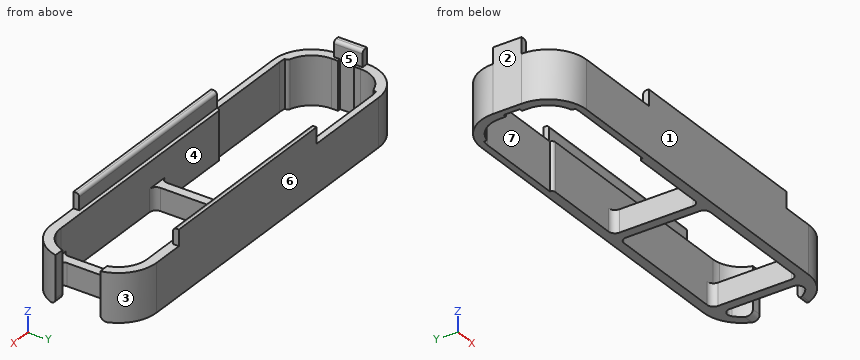
from build123d import *

# Parameters (mm, degrees)
BOSS_EXTRUDE2_DEPTH                    = 15
SKETCH4_W                              = 3
SKETCH4_H                              = 27
BOSS_EXTRUDE4_CROSS_STRUCTURES_DEPTH   = 15
SKETCH6_W                              = 3
SKETCH6_H                              = 27
CUT_EXTRUDE3_8_MM_SPACING_DEPTH        = 8
CUT_EXTRUDE4_ELECTRONICS_SPACING_DEPTH = 125.021167548
SKETCH8_W                              = 15
SKETCH8_H                              = 14
CUT_EXTRUDE2_USB_C_CUTOUT_DEPTH        = 5
FILLET2_USBC_R                         = 2
FILLET3_INNER_CORNERS_FRONT_R          = 1
FILLET5_INNER_CORNERS_R                = 2
SKETCH18_W                             = 62
SKETCH18_H                             = 1.8
SKETCH18_W_2                           = 2
SKETCH18_H_2                           = 9
BOSS_EXTRUDE7_DEPTH                    = 5
FILLET1_R                              = 1
SKETCH19_W                             = 1
SKETCH19_H                             = 5
CUT_EXTRUDE1_DEPTH                     = 124.762162398


with BuildPart() as part:
    # Sketch3 → Boss-Extrude2 (new body)
    with BuildSketch(Plane.XY.offset(-1.6194024)):
        with BuildLine():
            Line((110, 16.5), (10, 16.5))
            ThreePointArc((10, 16.5), (1.514718626, 12.985281374), (-2, 4.5))
            Line((-2, 4.5), (-2, -4.5))
            ThreePointArc((-2, -4.5), (1.514718626, -12.985281374), (10, -16.5))
            Line((10, -16.5), (110, -16.5))
            ThreePointArc((110, -16.5), (118.485281374, -12.985281374), (122, -4.5))
            Line((122, -4.5), (122, 4.5))
            ThreePointArc((122, 4.5), (118.485281374, 12.985281374), (110, 16.5))
        make_face()
        with BuildLine():
            Line((119, -4.5), (119, 4.5))
            ThreePointArc((119, 4.5), (116.363961031, 10.863961031), (110, 13.5))
            Line((110, 13.5), (10, 13.5))
            ThreePointArc((10, 13.5), (3.636038969, 10.863961031), (1, 4.5))
            Line((1, 4.5), (1, -4.5))
            ThreePointArc((1, -4.5), (3.636038969, -10.863961031), (10, -13.5))
            Line((10, -13.5), (110, -13.5))
            ThreePointArc((110, -13.5), (116.363961031, -10.863961031), (119, -4.5))
        make_face(mode=Mode.SUBTRACT)
    extrude(amount=-BOSS_EXTRUDE2_DEPTH)

    # Sketch4 → Boss-Extrude4 - cross structures (add)
    with BuildSketch(Plane.XY.offset(-1.6194024)):
        with Locations((110.9, 0)):
            Rectangle(SKETCH4_W, SKETCH4_H)
        with Locations((66.5, 0)):
            Rectangle(SKETCH4_W, SKETCH4_H)
    extrude(amount=-BOSS_EXTRUDE4_CROSS_STRUCTURES_DEPTH)

    # Sketch6 → Cut-Extrude3 - 8 mm spacing (cut)
    with BuildSketch(Plane.XY.offset(-1.6194024)):
        with BuildLine():
            Line((109.4, 13.5), (110, 13.5))
            ThreePointArc((110, 13.5), (111.211013131, 13.418152678), (112.4, 13.174099377))
            Line((112.4, 13.174099377), (112.4, -13.174099377))
            ThreePointArc((112.4, -13.174099377), (111.211013131, -13.418152678), (110, -13.5))
            Line((110, -13.5), (109.4, -13.5))
            Line((109.4, -13.5), (109.4, 13.5))
        make_face()
        with Locations((66.5, 0)):
            Rectangle(SKETCH6_W, SKETCH6_H)
    extrude(amount=-CUT_EXTRUDE3_8_MM_SPACING_DEPTH, mode=Mode.SUBTRACT)

    # Sketch7 → Cut-Extrude4 - electronics spacing (cut, through all)
    with BuildSketch(Plane.XY.offset(-1.6194024)):
        with BuildLine():
            Line((38, -14.5), (10, -14.5))
            ThreePointArc((10, -14.5), (8.99491038, -14.44936153), (8, -14.297958971))
            Line((8, -14.297958971), (8, 14.297958971))
            ThreePointArc((8, 14.297958971), (8.99491038, 14.44936153), (10, 14.5))
            Line((10, 14.5), (38, 14.5))
            Line((38, 14.5), (38, -14.5))
        make_face()
    extrude(amount=-CUT_EXTRUDE4_ELECTRONICS_SPACING_DEPTH, mode=Mode.SUBTRACT)

    # Sketch8 → Cut-Extrude2 - USB-C cutout (cut)
    with BuildSketch(Plane(origin=(122, 0, 0), x_dir=(0, 0, -1), z_dir=(1, 0, 0))):
        with Locations((9.1194024, 0)):
            Rectangle(SKETCH8_W, SKETCH8_H)
    extrude(amount=-CUT_EXTRUDE2_USB_C_CUTOUT_DEPTH, mode=Mode.SUBTRACT)

    # Fillet2 - USBC
    fillet2_usbc_edges = [part.edges().sort_by_distance(p)[0] for p in [
        (120.191251414, 7, -16.6194024),
        (120.191251414, -7, -16.6194024),
    ]]
    fillet(fillet2_usbc_edges, radius=FILLET2_USBC_R)

    # Fillet3 - inner corners, front
    fillet3_inner_corners_front_edges = [part.edges().sort_by_distance(p)[0] for p in [
        (38, 13.5, -9.1194024),
        (38, -13.5, -9.1194024),
        (8, -13.274964387, -9.1194024),
        (8, 13.274964387, -9.1194024),
    ]]
    fillet(fillet3_inner_corners_front_edges, radius=FILLET3_INNER_CORNERS_FRONT_R - 0.0001)  # a hair under: the kernel refuses the full size

    # Fillet5 - inner corners
    fillet5_inner_corners_edges = [part.edges().sort_by_distance(p)[0] for p in [
        (112.4, -13.174099377, -13.1194024),
        (109.4, -13.5, -13.1194024),
        (109.4, 13.5, -13.1194024),
        (65, -13.5, -13.1194024),
        (65, 13.5, -13.1194024),
        (68, 13.5, -13.1194024),
        (68, -13.5, -13.1194024),
        (112.4, 13.174099377, -13.1194024),
    ]]
    fillet(fillet5_inner_corners_edges, radius=FILLET5_INNER_CORNERS_R)

    # Sketch18 → Boss-Extrude7 (add)
    with BuildSketch(Plane.XY.offset(-1.6194024)):
        with Locations((69, 15.6)):
            Rectangle(SKETCH18_W, SKETCH18_H)
        with Locations((69, -15.6)):
            Rectangle(SKETCH18_W, SKETCH18_H)
        with Locations((-1, 0)):
            Rectangle(SKETCH18_W_2, SKETCH18_H_2)
    extrude(amount=BOSS_EXTRUDE7_DEPTH)

    # Fillet1
    fillet1_edges = [part.edges().sort_by_distance(p)[0] for p in [
        (69, 14.7, 3.3805976),
        (69, -14.7, 3.3805976),
        (0, 0, 3.3805976),
    ]]
    fillet(fillet1_edges, radius=FILLET1_R)

    # Sketch19 → Cut-Extrude1 (cut, through all)
    with BuildSketch(Plane.XY.offset(-1.6194024)):
        with Locations((0.5, 0)):
            Rectangle(SKETCH19_W, SKETCH19_H)
    extrude(amount=-CUT_EXTRUDE1_DEPTH, mode=Mode.SUBTRACT)


solid = part.part
Design review of the part built by this model. Coordinates are the model's own, in mm. Face numbers are marked on the shaded views. A direction names the side the tool comes from. Give positions to 0.01 mm unless a question says otherwise; leave off trailing zeros. Write each loop counter-clockwise with the first axis right and the second up, starting at its lowest first coordinate (ties: lowest second). Pieces come first, ordered by that corner, then holes. Notation, with made-up numbers: M -14,79 L -7,79 A22 ccw -7,98 Z; hole C -28.75,77 d11. An arc over 180 degrees is marked long. Return JSON: item names as keys, results as strings. Group by question number.
Item 1: Take a section at D-D (x = 106). Give the boundary of the cut face in (y, z).
Item 2: Take a section at A-A (x = 24). Give the boundary of the cut face in (y, z).
Item 3: The part is to be moulded in two halves that separate along X. For the marked faces 1, 2, 3 and 4, say which applies: pulls with the +X half, pulls with the -X half, needs draft (parallel to the pull), parting line crosses it, or undercut.
Item 4: Wall thickness on line 1 along X through (y, z) = (0, -12); line 2 along X through (y, z) = (4, -15.25); line 3 along Y through (x, z) = (86, -5): over which ranges is each line inside the solid? List them lowest first.
Item 5: Tool access review of the marked faces 5, 6 and 7: name each direction out of +Z, -Z, +X, -X, +Y, -Y from which nothing blocks a thin tool from reaching the whole face with its end or side.
Item 6: Take a section at B-B (z = 1.25). Give the boundary of the cut face in (x, y).
Item 7: Clearance check with flat-ended pins moving along their axes: pin 1 Ø7 at (x, y) = (34.5, 11.5) entering from +Z; pin 2 Ø3.5 at (x, y) = (67, -3.5) entering from +Z; pin 3 Ø1.4 at (y, z) = (15.5, 1) entering from +X. State where each tip first meets the part, or that it passes through.
Return value:
{
 "1": {"outline": "M -16.5,-16.62 L -13.5,-16.62 L -13.5,-1.62 L -16.5,-1.62 Z; M 13.5,-16.62 L 16.5,-16.62 L 16.5,-1.62 L 13.5,-1.62 Z"},
 "2": {"outline": "M -16.5,-16.62 L -14.5,-16.62 L -14.5,-1.62 L -16.5,-1.62 Z; M 14.5,-16.62 L 16.5,-16.62 L 16.5,-1.62 L 14.5,-1.62 Z"},
 "3": {"face 1": "needs draft", "face 2": "pulls with the -X half", "face 3": "pulls with the +X half", "face 4": "undercut"},
 "4": {"line 1": "x = -2 to 0, 65 to 68, 109.4 to 112.4", "line 2": "x = -2 to 1, 65 to 68, 109.4 to 112.4", "line 3": "y = -16.5 to -13.5, 13.5 to 16.5"},
 "5": {"face 5": "+Z", "face 6": "+Z, -Z, +X, -X, +Y", "face 7": "+Z, -Z"},
 "6": {"outline": "M -2,-4.5 L 0,-4.5 L 0,4.5 L -2,4.5 Z; M 38,-16.5 L 100,-16.5 L 100,-14.7 L 38,-14.7 Z; M 38,14.7 L 100,14.7 L 100,16.5 L 38,16.5 Z"},
 "7": {"pin 1": "stops at z = -1.62", "pin 2": "stops at z = -9.62", "pin 3": "stops at x = 100"}
}
